```python
from build123d import *

# Parameters (mm, degrees)
EXTRUDE_1_DEPTH     = 20
EXTRUDE_2_DEPTH     = 250
SKETCH_3_R          = 2.5
CUT_EXTRUDE_1_DEPTH = 250
SKETCH_4_R          = 5
CUT_EXTRUDE_2_DEPTH = 1500


with BuildPart() as part:
    # Эскиз1 → Бобышка-Вытянуть1 (new body)
    with BuildSketch(Plane(origin=(0, 0, 0), x_dir=(1, 0, 0), z_dir=(0, 1, 0))):
        with BuildLine():
            Line((-700, -650), (700, -650))
            ThreePointArc((700, -650), (735.355339059, -635.355339059), (750, -600))
            Line((750, -600), (750, 600))
            ThreePointArc((750, 600), (735.355339059, 635.355339059), (700, 650))
            Line((700, 650), (-700, 650))
            ThreePointArc((-700, 650), (-735.355339059, 635.355339059), (-750, 600))
            Line((-750, 600), (-750, -600))
            ThreePointArc((-750, -600), (-735.355339059, -635.355339059), (-700, -650))
        make_face()
    extrude(amount=EXTRUDE_1_DEPTH)

    # Эскиз2 → Бобышка-Вытянуть2 (add)
    with BuildSketch(Plane(origin=(0, 20, 0), x_dir=(1, 0, 0), z_dir=(0, 1, 0))):
        with BuildLine():
            Line((700, -650), (-700, -650))
            ThreePointArc((-700, -650), (-735.355339059, -635.355339059), (-750, -600))
            Line((-750, -600), (-750, 600))
            ThreePointArc((-750, 600), (-735.355339059, 635.355339059), (-700, 650))
            Line((-700, 650), (700, 650))
            ThreePointArc((700, 650), (735.355339059, 635.355339059), (750, 600))
            Line((750, 600), (750, -600))
            ThreePointArc((750, -600), (735.355339059, -635.355339059), (700, -650))
        make_face()
        with BuildLine():
            Line((665.384615385, -620), (-665.384615385, -620))
            ThreePointArc((-665.384615385, -620), (-700.739954444, -605.355339059), (-715.384615385, -570))
            Line((-715.384615385, -570), (-715.384615385, 570))
            ThreePointArc((-715.384615385, 570), (-700.739954444, 605.355339059), (-665.384615385, 620))
            Line((-665.384615385, 620), (665.384615385, 620))
            ThreePointArc((665.384615385, 620), (700.739954444, 605.355339059), (715.384615385, 570))
            Line((715.384615385, 570), (715.384615385, -570))
            ThreePointArc((715.384615385, -570), (700.739954444, -605.355339059), (665.384615385, -620))
        make_face(mode=Mode.SUBTRACT)
    extrude(amount=EXTRUDE_2_DEPTH)

    # Эскиз3 → Вырез-Вытянуть1 (cut)
    with BuildSketch(Plane.XZ):
        with Locations(Location((-650, -565, 0), (0, 0, 270))):
            Circle(SKETCH_3_R)
        with Locations(Location((-650, 565, 0), (0, 0, 270))):
            Circle(SKETCH_3_R)
        with Locations(Location((-665, 550, 0), (0, 0, 270))):
            Circle(SKETCH_3_R)
        with Locations(Location((-635, 550, 0), (0, 0, 270))):
            Circle(SKETCH_3_R)
        with Locations(Location((-650, 535, 0), (0, 0, 270))):
            Circle(SKETCH_3_R)
        with Locations(Location((665, 550, 0), (0, 0, 270))):
            Circle(SKETCH_3_R)
        with Locations(Location((650, 565, 0), (0, 0, 270))):
            Circle(SKETCH_3_R)
        with Locations(Location((635, 550, 0), (0, 0, 270))):
            Circle(SKETCH_3_R)
        with Locations(Location((650, 535, 0), (0, 0, 270))):
            Circle(SKETCH_3_R)
        with Locations(Location((650, -535, 0), (0, 0, 270))):
            Circle(SKETCH_3_R)
        with Locations(Location((635, -550, 0), (0, 0, 270))):
            Circle(SKETCH_3_R)
        with Locations(Location((665, -550, 0), (0, 0, 270))):
            Circle(SKETCH_3_R)
        with Locations(Location((650, -565, 0), (0, 0, 270))):
            Circle(SKETCH_3_R)
        with Locations(Location((-650, -535, 0), (0, 0, 270))):
            Circle(SKETCH_3_R)
        with Locations(Location((-665, -550, 0), (0, 0, 270))):
            Circle(SKETCH_3_R)
        with Locations(Location((-635, -550, 0), (0, 0, 270))):
            Circle(SKETCH_3_R)
    extrude(amount=-CUT_EXTRUDE_1_DEPTH, mode=Mode.SUBTRACT)

    # Эскиз4 → Вырез-Вытянуть2 (cut)
    with BuildSketch(Plane(origin=(0, 0, -650), x_dir=(-1, 0, 0), z_dir=(0, 0, -1))):
        with Locations((660, 260)):
            Circle(SKETCH_4_R)
    cut_extrude_2 = extrude(amount=-CUT_EXTRUDE_2_DEPTH, mode=Mode.SUBTRACT)

    # Зеркальное отражение1: Вырез-Вытянуть2 across plane
    add(cut_extrude_2.mirror(Plane.ZY), mode=Mode.SUBTRACT)


solid = part.part
```
Verification items for the finished model (mm, model axes). A direction names the side the tool comes from. Coordinates: 2 decimals unless noted, no trailing zeros. Loops run counter-clockwise (first coordinate to the right, second up) from the corner with the lowest first, then second, coordinate; pieces in that order, holes last. Notation, with made-up numbers: (72.25, -38.75) -> (101.25, -38.75) arc R20 cw to (101.25, -10.75) -> close; hole circle Ø2 at (-37.5, 10.5). An arc over 180 degrees is marked (long way). Answer in a Markdown table with one row per item. Add a question column.
1. Section check C-C, the plane x = -3.5. Enter the section's corners in (y, z).
2. Material ranges on probe 1 along X at (y, z) = (16, 550); probe 2 along X at (y, z) = (5.5, 535); probe 3 along Z at (x, y) = (-635, 6.25), recorded low to high. Write a range as [from, to].
3. Depth check by flat-ended pin: P1, Ø3, axis at x = -43, z = 225.5, coming from the +Y side. Enter the tip coordinate at first touch or a pass-through.
4. Access from +Z, -Z, +X, -X, +Y, -Y to the whole of each face (thin tool, end or side, straight path). Record for faces 5 (the face through (715.385, 143, -8)), 6 (the face through (-735.742, 133.11, -634.964)).
5. Section check B-B, the plane z = 269.5. Enter the section's corners in (x, y), then the cut area to 3 significant figures.
6. Draft check along X on faces 1 (the face through (735.742, 133.11, 634.964)), 2 (the face through (-750, 133, 8)), 3 (the face through (-10, 133, -650)), 4 (the face through (701.13, 143.25, 604.96)). Enter one of: +X half, -X half, draft (parallel to the pull), parting line (faces both ways), or undercut.
7. Section check A-A, the plane y = 43. Enter the section's corners in (x, z).
Derived:
| question | item | result |
|---|---|---|
| 1 | outline | (0, -650) -> (270, -650) -> (270, -620) -> (20, -620) -> (20, 620) -> (270, 620) -> (270, 650) -> (0, 650) -> close |
| 2 | probe 1 | x = [-750, -667.5], [-662.5, -637.5], [-632.5, 632.5], [637.5, 662.5], [667.5, 750] |
| 2 | probe 2 | x = [-750, -652.5], [-647.5, 647.5], [652.5, 750] |
| 2 | probe 3 | z = [-650, -552.5], [-547.5, 547.5], [552.5, 650] |
| 3 | P1 | stops at y = 20 |
| 4 | face 5 | +Y |
| 4 | face 6 | -Z, -X, +Y, -Y |
| 5 | outline | (-750, 0) -> (750, 0) -> (750, 270) -> (715.38, 270) -> (715.38, 20) -> (-715.38, 20) -> (-715.38, 270) -> (-750, 270) -> close |
| 5 | area | 47,300 mm² |
| 6 | face 1 | +X half |
| 6 | face 2 | -X half |
| 6 | face 3 | draft |
| 6 | face 4 | undercut |
| 7 | outline | (-750, -600) arc R50 ccw to (-700, -650) -> (700, -650) arc R50 ccw to (750, -600) -> (750, 600) arc R50 ccw to (700, 650) -> (-700, 650) arc R50 ccw to (-750, 600) -> close; hole (-715.38, -570) arc R50 ccw to (-665.38, -620) -> (665.38, -620) arc R50 ccw to (715.38, -570) -> (715.38, 570) arc R50 ccw to (665.38, 620) -> (-665.38, 620) arc R50 ccw to (-715.38, 570) -> close |
